from build123d import *

# Parameters (mm, degrees)
SKETCH1_W                      = 63.5
SKETCH1_H                      = 63.5
BOSS_EXTRUDE1_DEPTH            = 3.175
CBORE_FOR_M3_SHCS1_D           = 3.4
CBORE_FOR_M3_SHCS1_CBORE_D     = 6.5
CBORE_FOR_M3_SHCS1_CBORE_DEPTH = 3
M5_CLEARANCE_HOLE1_D           = 5.5
FILLET1_R                      = 3.175


with BuildPart() as part:
    # Sketch1 → Boss-Extrude1 (new, symmetric)
    with BuildSketch(Plane.XY):
        Rectangle(SKETCH1_W, SKETCH1_H)
    extrude(amount=BOSS_EXTRUDE1_DEPTH, both=True)

    # CBORE for M3 SHCS1 (through all)
    with Locations(Plane.XY.offset(3.175)):
        with Locations((-10, -10), (10, 10), (-10, 10), (10, -10)):
            CounterBoreHole(CBORE_FOR_M3_SHCS1_D / 2, CBORE_FOR_M3_SHCS1_CBORE_D / 2, CBORE_FOR_M3_SHCS1_CBORE_DEPTH)

    # M5 Clearance Hole1 (through all)
    with Locations(Plane.XY.offset(3.175)):
        with Locations((-25.4, -25.4), (-25.4, 25.4), (25.4, -25.4), (25.4, 25.4)):
            Hole(M5_CLEARANCE_HOLE1_D / 2)

    # Fillet1
    fillet1_edges = [part.edges().sort_by_distance(p)[0] for p in [
        (-31.75, 31.75, 0),
        (31.75, 31.75, 0),
        (31.75, -31.75, 0),
        (-31.75, -31.75, 0),
    ]]
    fillet(fillet1_edges, radius=FILLET1_R)


solid = part.part
Read the model definition and answer for the solid it produces. Units are mm, in the model's axes. A direction names the side the tool comes from. Coordinates: 2 decimals unless noted, no trailing zeros. Order: outer loops, then holes, each group sorted by start corner. A loop starts at its lowest first (then second) coordinate and runs counter-clockwise, first axis right, second up. Notation, with made-up numbers: M 78.5,7.25 L 129.5,7.25 A22 ccw 129.5,22.25 Z; hole C 70,32 d2. An arc over 180 degrees is marked long. Put each result on its own line as item: value. Start each with the question number.
Item 1: Consider probe 1 along Y at (x, z) = (10, -1.55); probe 2 along Y at (x, z) = (-25.4, 1.5); probe 3 along X at (y, z) = (25, -1.75). Determine where each line is inside the solid, lowest interval first. Write a range as [from, to].
Item 2: Section C-C, the plane z = 2 is taken. Count the separate pieces of the cut face and the enclosed holes in it, plus the area to 3 significant figures.
Item 3: The mould has two halves that part along Y. Classify faces 1 (the face through (-30.84, -30.8, 0.04)), 2 (the face through (24.13, -27.84, -0.04)), 3 (the face through (-31.75, 0, 0)): +Y half, -Y half, draft (parallel to the pull), parting line (faces both ways), or undercut.
Item 4: For faces 4 (the face through (-9.63, -11.66, -1.52)), 5 (the face through (-12.395, 12.197, 1.696)), determine the directions among +Z, -Z, +X, -X, +Y, -Y from which every point of the face is accessible in a straight line to the end or side of a thin tool.
Item 5: Section D-D, the plane x = 25.4 is taken. Determine the outline of the cut face in (y, z) (3 decimals).
Item 6: Section A-A, the plane x = 10 is taken. Determine the outline of the cut face in (y, z) (3 decimals), plus the area to 3 significant figures.
Computed:
1. probe 1: y = [-31.75, -11.7], [-8.3, 8.3], [11.7, 31.75]
1. probe 2: y = [-31.75, -28.15], [-22.65, 22.65], [28.15, 31.75]
1. probe 3: x = [-31.75, -28.12], [-22.68, 22.68], [28.12, 31.75]
2. separate pieces: 1
2. enclosed holes: 8
2. area: 3,800 mm2
3. face 1: -Y half
3. face 2: undercut
3. face 3: draft
4. face 4: +Z, -Z
4. face 5: +Z
5. outline: M -31.75,-3.175 L -28.15,-3.175 L -28.15,3.175 L -31.75,3.175 Z; M -22.65,-3.175 L 22.65,-3.175 L 22.65,3.175 L -22.65,3.175 Z; M 28.15,-3.175 L 31.75,-3.175 L 31.75,3.175 L 28.15,3.175 Z
6. outline: M -31.75,-3.175 L -11.7,-3.175 L -11.7,0.175 L -13.25,0.175 L -13.25,3.175 L -31.75,3.175 Z; M -8.3,-3.175 L 8.3,-3.175 L 8.3,0.175 L 6.75,0.175 L 6.75,3.175 L -6.75,3.175 L -6.75,0.175 L -8.3,0.175 Z; M 11.7,-3.175 L 31.75,-3.175 L 31.75,3.175 L 13.25,3.175 L 13.25,0.175 L 11.7,0.175 Z
6. area: 341 mm2
